Model file for the job. Use its own axes, mm. A direction names the side the tool comes from. Round coordinates to 2 decimals unless told otherwise and drop trailing zeros. Loops run counter-clockwise (first coordinate to the right, second up) from the corner with the lowest first, then second, coordinate; pieces in that order, holes last. Notation, with made-up numbers: M 74,33 L 132,33 A18 ccw 132,45 Z; hole C 77.5,-23 d6. An arc over 180 degrees is marked long. Use a Markdown table: item, result. Add a question column.
Item 1: Two-plate mould, pull along X, no slides. Class faces 1 (the flat face through (6.5, -39, 1)), 2 (the cylindrical face through (-5.6, -52.64, 1.52)), 3 (the cylindrical face through (-0.595, -16.456, 1.521)), 4 (the flat face through (0, -21, 3)): +X half, -X half, draft (parallel to the pull), parting line (faces both ways), or undercut.
Item 2: Saw through at B-B on z = 1.7. Write the cut outline in (x, y), then the cut area to 3 significant figures.
Item 3: Saw through at A-A on y = -31.5. Write the cut outline in (x, z), then the cut area to 3 significant figures.
Item 4: Tool access for faces 5 (the flat face through (-1.55, -45, 2)), 6 (the flat face through (-6.5, -38, 1)), 7 (the flat face through (0, -53.5, 1)): list every direction of +Z, -Z, +X, -X, +Y, -Y with a clear straight run to the whole face (end or side of a thin tool).
Item 5: Wall check: L1, parallel to Y at x = 0, z = 1.75; L2, parallel to X at y = -43.5, z = 2.4; L3, parallel to X at y = -31, z = 0.25. Give the ranges that are in metal, low to high. Write a range as from..to.
Item 6: Saw through at C-C on y = -16. Write the cut outline in (x, z), then the cut area to 3 significant figures.
Item 7: Saw through at D-D on x = -7.25. Write the cut outline in (y, z).
Item 8: Pin check, flat tips, straight feed: P1, Ø6, axis at x = 0, y = 0, coming from the -Z side; P2, Ø0.9, axis at x = 0, y = -16, coming from the -Z side; P3, Ø0.9, axis at y = -44.5, z = 2, coming from the +X side. Stop position of each tip, or through.
```python
from build123d import *

# Parameters (mm, degrees)
SALIENTE_EXTRUIR1_DEPTH = 3
CROQUIS2_R              = 2.5
CROQUIS2_R_2            = 1.5
CROQUIS2_W              = 3.1
CROQUIS2_H              = 7
CORTAR_EXTRUIR1_DEPTH   = 3
REDONDEO1_R             = 60
REDONDEO2_R             = 3
CROQUIS3_R              = 0.75
CORTAR_EXTRUIR2_DEPTH   = 3


with BuildPart() as part:
    # Croquis1 → Saliente-Extruir1 (new body)
    with BuildSketch(Plane.XY):
        with BuildLine():
            Line((-6.5, -53.5), (6.5, -53.5))
            Line((6.5, -53.5), (6.5, -9.486832981))
            ThreePointArc((6.5, -9.486832981), (0, -11.5), (-6.5, -9.486832981))
            Line((-6.5, -9.486832981), (-6.5, -53.5))
        make_face()
        with BuildLine():
            ThreePointArc((-6.5, -9.486832981), (0, -11.5), (6.5, -9.486832981))
            Line((6.5, -9.486832981), (6.5, 0))
            Line((6.5, 0), (-6.5, 0))
            Line((-6.5, 0), (-6.5, -9.486832981))
        make_face()
        with BuildLine():
            Line((6.5, 0), (6.5, -9.486832981))
            ThreePointArc((6.5, -9.486832981), (10.173494975, -5.361902647), (11.5, 0))
            ThreePointArc((11.5, 0), (-5.361902647, 10.173494975), (-6.5, -9.486832981))
            Line((-6.5, -9.486832981), (-6.5, 0))
            Line((-6.5, 0), (6.5, 0))
        make_face()
    extrude(amount=SALIENTE_EXTRUIR1_DEPTH)

    # Croquis2 → Cortar-Extruir1 (cut)
    with BuildSketch(Plane.XY.offset(3)):
        Circle(CROQUIS2_R)
        with Locations((0, -31.5)):
            Circle(CROQUIS2_R_2)
        with Locations((0, -45)):
            Rectangle(CROQUIS2_W, CROQUIS2_H)
    extrude(amount=-CORTAR_EXTRUIR1_DEPTH, mode=Mode.SUBTRACT)

    # Redondeo1
    redondeo1_edges = [part.edges().sort_by_distance(p)[0] for p in [
        (-6.5, -9.486832981, 1.5),
        (6.5, -9.486832981, 1.5),
    ]]
    fillet(redondeo1_edges, radius=REDONDEO1_R)

    # Redondeo2
    redondeo2_edges = [part.edges().sort_by_distance(p)[0] for p in [
        (6.5, -53.5, 1.5),
        (-6.5, -53.5, 1.5),
    ]]
    fillet(redondeo2_edges, radius=REDONDEO2_R)

    # Croquis3 → Cortar-Extruir2 (cut)
    with BuildSketch(Plane.XY.offset(3)):
        with Locations((0, 8)):
            Circle(CROQUIS3_R)
        with Locations((0, -16)):
            Circle(CROQUIS3_R)
    extrude(amount=-CORTAR_EXTRUIR2_DEPTH, mode=Mode.SUBTRACT)


solid = part.part
```
Entries:
| question | item | result |
|---|---|---|
| 1 | face 1 | +X half |
| 1 | face 2 | -X half |
| 1 | face 3 | undercut |
| 1 | face 4 | draft |
| 2 | outline | M -10.7,-4.22 A60 cw -6.5,-26.27 L -6.5,-50.5 A3 ccw -3.5,-53.5 L 3.5,-53.5 A3 ccw 6.5,-50.5 L 6.5,-26.27 A60 cw 10.7,-4.22 A11.5 ccw long Z; hole C 0,0 d5; hole M -1.55,-48.5 L 1.55,-48.5 L 1.55,-41.5 L -1.55,-41.5 Z; hole C 0,-31.5 d3; hole C 0,-16 d1.5; hole C 0,8 d1.5 |
| 2 | area | 948 mm2 |
| 3 | outline | M -6.5,0 L -1.5,0 L -1.5,3 L -6.5,3 Z; M 1.5,0 L 6.5,0 L 6.5,3 L 1.5,3 Z |
| 3 | area | 30.0 mm2 |
| 4 | face 5 | +Z, -Z |
| 4 | face 6 | +Z, -Z, -X, -Y |
| 4 | face 7 | +Z, -Z, +X, -X, -Y |
| 5 | L1 | -53.5..-48.5, -41.5..-33, -30..-16.75, -15.25..-2.5, 2.5..7.25, 8.75..11.5 |
| 5 | L2 | -6.5..-1.55, 1.55..6.5 |
| 5 | L3 | -6.5..-1.41, 1.41..6.5 |
| 6 | outline | M -7.39,0 L -0.75,0 L -0.75,3 L -7.39,3 Z; M 0.75,0 L 7.39,0 L 7.39,3 L 0.75,3 Z |
| 6 | area | 39.8 mm2 |
| 7 | outline | M -16.81,0 L 8.93,0 L 8.93,3 L -16.81,3 Z |
| 8 | P1 | z = 0 |
| 8 | P2 | through |
| 8 | P3 | x = 6.5 |
